Geometry check sheet. Reference: the model listing, model coordinates, mm. Round coordinates to 2 decimals unless told otherwise and drop trailing zeros. Order: outer loops, then holes, each group sorted by start corner. A loop starts at its lowest first (then second) coordinate and runs counter-clockwise, first axis right, second up. Notation, with made-up numbers: M -5,-29.5 L 26,-29.5 A18 ccw 26,-12.5 Z; hole C 6,56.25 d1. An arc over 180 degrees is marked long. Return JSON: item names as keys, results as strings. Group by question number.
```python
from build123d import *

# Parameters (mm, degrees)
F0_R     = 3.175
F0_R_2   = 3.2155850094
F1_DEPTH = 3.048


with BuildPart() as f1:
    # F0 (on Top) → F1 (new body)
    with BuildSketch(Plane.XY):
        with BuildLine():
            ThreePointArc((20.8380485389, 43.6243366756), (20.8460123248, 43.8490943624), (20.8486674135, 44.0739774213))
            ThreePointArc((20.8486674135, 44.0739774213), (20.7075310622, 45.7076016198), (20.2883045743, 47.2928134805))
            Line((20.2883045743, 47.2928134805), (20.8380485389, 43.6243366756))
        make_face()
        with BuildLine():
            Line((20.8380485389, 43.6243366756), (20.2883045743, 47.2928134805))
            ThreePointArc((20.2883045743, 47.2928134805), (11.4947007425, 53.5974417385), (2.4803889816, 47.6126285169))
            Line((2.4803889816, 47.6126285169), (1.8290711011, 43.3135394793))
            ThreePointArc((1.8290711011, 43.3135394793), (11.4793805601, 34.5502502929), (20.8380485389, 43.6243366756))
        make_face()
        with Locations((11.3236674135, 44.0739774213)):
            Circle(F0_R, mode=Mode.SUBTRACT)
        with BuildLine():
            Line((27.0228593645, 2.3526965767), (20.8380485389, 43.6243366756))
            ThreePointArc((20.8380485389, 43.6243366756), (11.4793805601, 34.5502502929), (1.8290711011, 43.3135394793))
            Line((1.8290711011, 43.3135394793), (-4.3727269733, 2.3779488711))
            ThreePointArc((-4.3727269733, 2.3779488711), (11.3359323796, 15.8749948649), (27.0228593645, 2.3526965767))
        make_face()
        with Locations((8.1481637045, 30.2663650364)):
            Circle(F0_R_2, mode=Mode.SUBTRACT)
        with BuildLine():
            Line((1.8290711011, 43.3135394793), (2.4803889816, 47.6126285169))
            ThreePointArc((2.4803889816, 47.6126285169), (1.9061330136, 45.5007467885), (1.8290711011, 43.3135394793))
        make_face()
        with BuildLine():
            Line((27.3754255146, 0), (27.0228593645, 2.3526965767))
            ThreePointArc((27.0228593645, 2.3526965767), (27.1542769566, 1.1796093414), (27.1981637045, 0))
            ThreePointArc((27.1981637045, 0), (10.1308213687, -15.8301593408), (-4.3727269733, 2.3779488711))
            Line((-4.3727269733, 2.3779488711), (-4.7329894859, 0))
            Line((-4.7329894859, 0), (1.8478131932, -64.4672828145))
            ThreePointArc((1.8478131932, -64.4672828145), (10.839303468, -53.9873184958), (20.8485711575, -63.5000000212))
            ThreePointArc((20.8485711575, -63.5000000212), (18.365147651, -69.9141894077), (12.2098676434, -72.9836756556))
            Line((12.2098676434, -72.9836756556), (56.0542108535, -71.4325372605))
            ThreePointArc((56.0542108535, -71.4325372605), (47.837920469, -63.6713312347), (55.7115808743, -55.5627420555))
            Line((55.7115808743, -55.5627420555), (30.2908926845, -54.6499382367))
            ThreePointArc((30.2908926845, -54.6499382367), (24.5800251587, -51.9251805627), (22.6674883506, -45.8935543113))
            Line((22.6674883506, -45.8935543113), (27.3754255146, 0))
        make_face()
        with BuildLine():
            ThreePointArc((27.1981637045, 0), (27.1542769566, 1.1796093414), (27.0228593645, 2.3526965767))
            ThreePointArc((27.0228593645, 2.3526965767), (11.3359323796, 15.8749948649), (-4.3727269733, 2.3779488711))
            ThreePointArc((-4.3727269733, 2.3779488711), (10.1308213687, -15.8301593408), (27.1981637045, 0))
        make_face()
        with Locations((11.3231637045, 0)):
            Circle(F0_R, mode=Mode.SUBTRACT)
        with BuildLine():
            ThreePointArc((20.8485711575, -63.5000000212), (10.839303468, -53.9873184958), (1.8478131932, -64.4672828145))
            ThreePointArc((1.8478131932, -64.4672828145), (5.2756831891, -70.8585784248), (12.2098676434, -72.9836756556))
            ThreePointArc((12.2098676434, -72.9836756556), (18.365147651, -69.9141894077), (20.8485711575, -63.5000000212))
        make_face()
        with Locations((11.3235711575, -63.5000000212)):
            Circle(F0_R, mode=Mode.SUBTRACT)
        with BuildLine():
            ThreePointArc((63.7110711578, -63.499999986), (61.364271399, -57.8654656607), (55.7115808743, -55.5627420555))
            ThreePointArc((55.7115808743, -55.5627420555), (47.837920469, -63.6713312347), (56.0542108535, -71.4325372605))
            ThreePointArc((56.0542108535, -71.4325372605), (61.4845904991, -69.0125460704), (63.7110711578, -63.499999986))
        make_face()
        with Locations((55.7735711578, -63.499999986)):
            Circle(F0_R, mode=Mode.SUBTRACT)
    extrude(amount=F1_DEPTH)


solid = f1.part
```
Q1. Depth check by flat-ended pin: pin 1 Ø1.5 at (y, z) = (-12, 1.5) entering from -X. Enter the tip coordinate at first touch or a pass-through.
Q2. Section check B-B on y = -34.5. Record the cut outline in (x, z).
Q3. Section check C-C on x = 17. Record the cut outline in (y, z), plus the area to 3 significant figures.
Q4. Section check A-A on z = 0.75. Count the separate pieces of the cut face and the enclosed holes in it, plus the area to 3 significant figures.
Q5. Release check for a two-part mould opening along X. For faces 1 (the face through (10.64, -66.6, 1.5)), 2 (the face through (13.03, 46.75, 1.5)), 3 (the face through (-1.49, -31.78, 1.5)), 4 (the face through (24.99, -23.27, 1.5)) record: +X half, -X half, draft (parallel to the pull), parting line (faces both ways), or undercut.
Q6. Material ranges on line 1 along Y through (x, z) = (10.5, 1.75); line 2 along Y through (x, z) = (9.5, 1.2); line 3 along Y through (x, z) = (12, 1.1), recorded low to high.
Geometry check:
{
 "1": {"pin 1": "stops at x = -3.58"},
 "2": {"outline": "M -1.21,0 L 23.84,0 L 23.84,3.05 L -1.21,3.05 Z"},
 "3": {"outline": "M -72.81,0 L 51.72,0 L 51.72,3.05 L -72.81,3.05 Z", "area": "380 mm^2"},
 "4": {"separate pieces": "1", "enclosed holes": "5", "area": "3,600 mm^2"},
 "5": {"face 1": "undercut", "face 2": "undercut", "face 3": "-X half", "face 4": "+X half"},
 "6": {"line 1": "y = -72.99 to -66.57, -60.43 to -3.07, 3.07 to 28.07, 32.46 to 41.01, 47.14 to 53.56", "line 2": "y = -72.85 to -66.1, -60.9 to -2.6, 2.6 to 27.35, 33.18 to 41.47, 46.67 to 53.42", "line 3": "y = -73 to -66.6, -60.4 to -3.1, 3.1 to 40.97, 47.18 to 53.57"}
}
